from build123d import *

# Parameters (mm, degrees)
ESQUISSE1_R             = 40
BOSS_EXTRU_2_DEPTH      = 35
ESQUISSE4_R             = 35
ENL_V_MAT_EXTRU_2_DEPTH = 18
ESQUISSE6_R             = 2.5
ENL_V_MAT_EXTRU_4_DEPTH = 12
ESQUISSE5_R             = 40
ENL_V_MAT_EXTRU_5_DEPTH = 12
ESQUISSE7_R             = 5
ENL_V_MAT_EXTRU_7_DEPTH = 10


with BuildPart() as part:
    # Esquisse1 → Boss.-Extru.2 (new body)
    with BuildSketch(Plane(origin=(0, 0, 0), x_dir=(1, 0, 0), z_dir=(0, 1, 0))):
        with Locations(Location((0, 0, 0), (0, 0, 270))):
            Circle(ESQUISSE1_R)
    extrude(amount=BOSS_EXTRU_2_DEPTH)

    # Esquisse4 → Enlèv. mat.-Extru.2 (cut)
    with BuildSketch(Plane(origin=(0, 35, 0), x_dir=(1, 0, 0), z_dir=(0, 1, 0))):
        with Locations(Location((0, 0, 0), (0, 0, 270))):
            Circle(ESQUISSE4_R)
    extrude(amount=-ENL_V_MAT_EXTRU_2_DEPTH, mode=Mode.SUBTRACT)

    # Esquisse6 → Enlèv. mat.-Extru.4 (cut)
    with BuildSketch(Plane(origin=(0, 17, 0), x_dir=(1, 0, 0), z_dir=(0, 1, 0))):
        with Locations(Location((0, 0, 0), (0, 0, 270))):
            Circle(ESQUISSE6_R)
    extrude(amount=-ENL_V_MAT_EXTRU_4_DEPTH, mode=Mode.SUBTRACT)

    # Esquisse5 → Enlèv. mat.-Extru.5 (cut)
    with BuildSketch(Plane(origin=(0, 0, 0), x_dir=(-1, 0, 0), z_dir=(0, -1, 0))):
        with Locations(Location((0, 0, 0), (0, 0, 90))):
            Circle(ESQUISSE5_R)
    extrude(amount=-ENL_V_MAT_EXTRU_5_DEPTH, mode=Mode.SUBTRACT)

    # Esquisse7 → Enlèv. mat.-Extru.7 (cut)
    with BuildSketch(Plane.XZ.offset(-12)):
        with Locations(Location((-25, 0, 0), (0, 0, 270))):
            Circle(ESQUISSE7_R)
        with Locations(Location((-17.67766953, 17.67766953, 0), (0, 0, 270))):
            Circle(ESQUISSE7_R)
        with Locations(Location((0, 25, 0), (0, 0, 270))):
            Circle(ESQUISSE7_R)
        with Locations(Location((17.67766953, 17.67766953, 0), (0, 0, 270))):
            Circle(ESQUISSE7_R)
        with Locations(Location((25, 0, 0), (0, 0, 270))):
            Circle(ESQUISSE7_R)
        with Locations(Location((17.67766953, -17.67766953, 0), (0, 0, 270))):
            Circle(ESQUISSE7_R)
        with Locations(Location((0, -25, 0), (0, 0, 270))):
            Circle(ESQUISSE7_R)
        with Locations(Location((-17.67766953, -17.67766953, 0), (0, 0, 270))):
            Circle(ESQUISSE7_R)
    extrude(amount=-ENL_V_MAT_EXTRU_7_DEPTH, mode=Mode.SUBTRACT)


solid = part.part
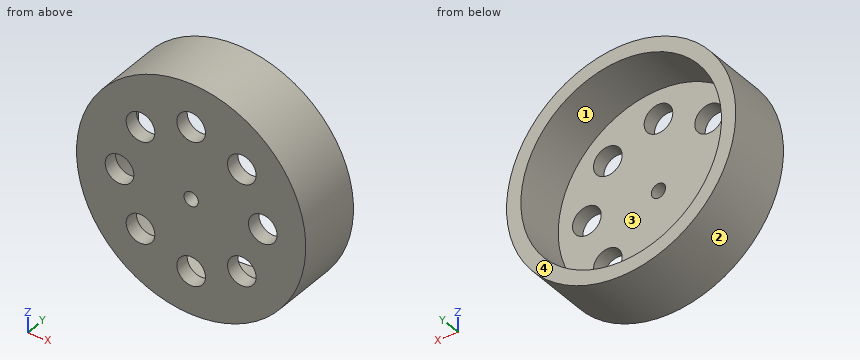
The model under review builds one solid part; all positions refer to its coordinate system, in mm. Face numbers are marked on the shaded views. Coordinates: 2 decimals unless noted, no trailing zeros. Loops run counter-clockwise (first coordinate to the right, second up) from the corner with the lowest first, then second, coordinate; pieces in that order, holes last. Notation, with made-up numbers: M -23,-11.5 L 16,-11.5 A33 cw 16,17.5 Z; hole C 87,48 d4. An arc over 180 degrees is marked long. Put each result on its own line as item: value. Start each with the question number.
Q1. Add section B-B (x = -25). Write out the cut boundary in (y, z).
Q2. Clearance check with flat-ended pins moving along their axes: pin 1 (8 mm diameter, centred on x = 25, z = 0, fed in from +Y); pin 2 (2 mm diameter, centred on x = 22.5, z = 19.5, fed in from +Y); pin 3 (10 mm diameter, centred on y = 15.5, z = -29, fed in from -X); pin 4 (2 mm diameter, centred on x = 11.5, y = 29.5, fed in from -Z). State where each tip first meets the part, or that it passes through.
Q3. Add section D-D (y = 14.25). Count the separate pieces of the cut face and the enclosed holes in it, and give its area (3 significant figures).
Q4. Add section A-A (z = 0). Write out the cut boundary in (x, y).
Q5. Add section C-C (x = -14). Write out the cut boundary in (y, z), and give its area (3 significant figures).
Q6. The part is to be moulded in two halves that separate along Z. For the marked faces 1, 2, 3 and 4, say which applies: +Z half, -Z half, draft (parallel to the pull), parting line (faces both ways), or undercut.
Q7. Wall thickness on line 1 (X direction, y = 30.75, z = 0); line 2 (Y direction, x = 34, z = -6); line 3 (Z direction, x = 19, y = 16): over which ranges is each line inside the solid? List them lowest first.
Answers:
1. outline: M 12,-31.22 L 35,-31.22 L 35,-24.49 L 17,-24.49 L 17,-5 L 12,-5 Z; M 12,5 L 17,5 L 17,24.49 L 35,24.49 L 35,31.22 L 12,31.22 Z
2. pin 1: passes through
2. pin 2: stops at y = 17
2. pin 3: stops at x = -32
2. pin 4: stops at z = -38.6
3. separate pieces: 1
3. enclosed holes: 9
3. area: 4,380 mm^2
4. outline: M -40,12 L -30,12 L -30,17 L -35,17 L -35,35 L -40,35 Z; M -20,12 L -2.5,12 L -2.5,17 L -20,17 Z; M 2.5,12 L 20,12 L 20,17 L 2.5,17 Z; M 30,12 L 40,12 L 40,35 L 35,35 L 35,17 L 30,17 Z
5. outline: M 12,-37.47 L 35,-37.47 L 35,-32.08 L 17,-32.08 L 17,-21.07 L 12,-21.07 Z; M 12,-14.29 L 17,-14.29 L 17,14.29 L 12,14.29 Z; M 12,21.07 L 17,21.07 L 17,32.08 L 35,32.08 L 35,37.47 L 12,37.47 Z
5. area: 501 mm^2
6. face 1: undercut
6. face 2: parting line
6. face 3: undercut
6. face 4: draft
7. line 1: x = -40 to -35, 35 to 40
7. line 2: y = 12 to 17
7. line 3: z = -35.2 to -22.5, -12.86 to 12.86, 22.5 to 35.2
